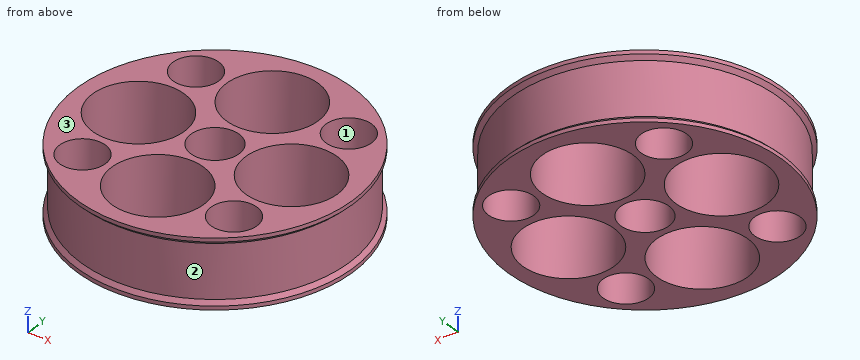
from build123d import *

# Parameters (mm, degrees)
F0_R     = 17.5
F0_R_2   = 3
F0_R_3   = 6
F0_R_4   = 3.15
F1_DEPTH = 7
F2_R     = 18
F2_R_2   = 17.5
F2_R_3   = 3
F2_R_4   = 6
F2_R_5   = 3.15
F3_DEPTH = 1
F4_R     = 18
F4_R_2   = 17.5
F4_R_3   = 3
F4_R_4   = 6
F4_R_5   = 3.15
F5_DEPTH = 1
F6_SIZE  = 0.49999


# Not quite as in the source:
# - a fillet or chamfer is up to 0.001 mm smaller than in the source, because OpenCascade refuses the exact size


with BuildPart() as f1:
    # F0 (on Top) → F1 (new body)
    with BuildSketch(Plane.XY):
        Circle(F0_R)
        with Locations((-9.8994949366, -9.8994949366)):
            Circle(F0_R_2, mode=Mode.SUBTRACT)
        with Locations((0, -10)):
            Circle(F0_R_3, mode=Mode.SUBTRACT)
        with Locations((9.8994949366, -9.8994949366)):
            Circle(F0_R_2, mode=Mode.SUBTRACT)
        with Locations((-10, 0)):
            Circle(F0_R_3, mode=Mode.SUBTRACT)
        with Locations((-9.8994949366, 9.8994949366)):
            Circle(F0_R_2, mode=Mode.SUBTRACT)
        Circle(F0_R_4, mode=Mode.SUBTRACT)
        with Locations((10, 0)):
            Circle(F0_R_3, mode=Mode.SUBTRACT)
        with Locations((0, 10)):
            Circle(F0_R_3, mode=Mode.SUBTRACT)
        with Locations((10, 10)):
            Circle(F0_R_2, mode=Mode.SUBTRACT)
    extrude(amount=F1_DEPTH)

    # F2 (on face) → F3 (join)
    with BuildSketch(Plane.XY.offset(7)):
        Circle(F2_R)
        Circle(F2_R_2, mode=Mode.SUBTRACT)
        Circle(F2_R_2)
        with Locations((-9.8994949366, -9.8994949366)):
            Circle(F2_R_3, mode=Mode.SUBTRACT)
        with Locations((0, -10)):
            Circle(F2_R_4, mode=Mode.SUBTRACT)
        with Locations((9.8994949366, -9.8994949366)):
            Circle(F2_R_3, mode=Mode.SUBTRACT)
        with Locations((-10, 0)):
            Circle(F2_R_4, mode=Mode.SUBTRACT)
        with Locations((-9.8994949366, 9.8994949366)):
            Circle(F2_R_3, mode=Mode.SUBTRACT)
        Circle(F2_R_5, mode=Mode.SUBTRACT)
        with Locations((10, 0)):
            Circle(F2_R_4, mode=Mode.SUBTRACT)
        with Locations((0, 10)):
            Circle(F2_R_4, mode=Mode.SUBTRACT)
        with Locations((10, 10)):
            Circle(F2_R_3, mode=Mode.SUBTRACT)
    extrude(amount=F3_DEPTH)

    # F4 (on face) → F5 (join)
    with BuildSketch(Plane(origin=(0, 0, 0), x_dir=(1, 0, 0), z_dir=(0, 0, -1))):
        Circle(F4_R)
        Circle(F4_R_2, mode=Mode.SUBTRACT)
        Circle(F4_R_2)
        with Locations((-9.8994949366, -9.8994949366)):
            Circle(F4_R_3, mode=Mode.SUBTRACT)
        with Locations((0, -10)):
            Circle(F4_R_4, mode=Mode.SUBTRACT)
        with Locations((10, -10)):
            Circle(F4_R_3, mode=Mode.SUBTRACT)
        with Locations((-10, 0)):
            Circle(F4_R_4, mode=Mode.SUBTRACT)
        with Locations((-9.8994949366, 9.8994949366)):
            Circle(F4_R_3, mode=Mode.SUBTRACT)
        Circle(F4_R_5, mode=Mode.SUBTRACT)
        with Locations((10, 0)):
            Circle(F4_R_4, mode=Mode.SUBTRACT)
        with Locations((0, 10)):
            Circle(F4_R_4, mode=Mode.SUBTRACT)
        with Locations((9.8994949366, 9.8994949366)):
            Circle(F4_R_3, mode=Mode.SUBTRACT)
    extrude(amount=F5_DEPTH)

    # F6 (size 0.5 in the source; OpenCascade refuses exactly that, so slightly less here)
    f6_edges = [f1.edges().sort_by_distance(p)[0] for p in [
        (-18, 0, 0),
        (-18, 0, 7),
    ]]
    chamfer(f6_edges, length=F6_SIZE)


solid = f1.part
Here's how the part is built. I have some questions about the finished solid (model axes, mm). Face numbers are marked on the shaded views. Round coordinates to 2 decimals unless told otherwise and drop trailing zeros. Return JSON: item names as keys, results as strings. Group by question number.
1. Please list where these lines run through material, in increasing order: probe 1 along Y at (x, z) = (0, 6.25); probe 2 along X at (y, z) = (9.5, 0.5); probe 3 along X at (y, z) = (-2, 1).
2. I'm going to push flat-ended pins straight in: pin 1 Ø11 at (x, y) = (0, 10) entering from -Z; pin 2 Ø5 at (y, z) = (-14, 6) entering from -X; pin 3 Ø2 at (x, z) = (6, 6) entering from -Y; pin 4 Ø5 at (y, z) = (-3.5, 7) entering from -X. Where does each tip first touch, or does it pass through?
3. If we section it at A-A on y = 0: State how many separate pieces and enclosed holes the cut face has, then the cut area to 3 significant figures.
4. If we mould it in two halves opening along X, with no side actions, what happens to the marked faces 1, 2 and 3? For each: pulls with the +X half, pulls with the -X half, needs draft (parallel to the pull), parting line crosses it, or undercut.
Reply:
{
 "1": {"probe 1": "-17.5 to -16, -4 to -3.15, 3.15 to 4, 16 to 17.5", "probe 2": "-14.7 to -12.87, -6.93 to -5.98, 5.98 to 7.04, 12.96 to 14.7", "probe 3": "-17.39 to -15.66, -4.34 to -2.43, 2.43 to 4.34, 15.66 to 17.39"},
 "2": {"pin 1": "through", "pin 2": "x = -13.42", "pin 3": "y = -16.77", "pin 4": "x = -17.97"},
 "3": {"separate pieces": "4", "enclosed holes": "0", "area": "43.8 mm^2"},
 "4": {"face 1": "undercut", "face 2": "parting line crosses it", "face 3": "needs draft"}
}
